from build123d import *

# Parameters (mm, degrees)
SKETCH1_W            = 914
SKETCH1_H            = 430
BOSS_EXTRUDE1_DEPTH  = 15
CUT_EXTRUDE2_DEPTH   = 16
LPATTERN1_COUNT      = 4
LPATTERN1_PITCH      = 80
MIRROR1_COPY_1_DEPTH = 16
MIRROR1_COPY_2_DEPTH = 16
MIRROR1_COPY_3_DEPTH = 16


with BuildPart() as part:
    # Sketch1 → Boss-Extrude1 (new body)
    with BuildSketch(Plane(origin=(0, 0, 0), x_dir=(1, 0, 0), z_dir=(0, 1, 0))):
        Rectangle(SKETCH1_W, SKETCH1_H)
    extrude(amount=BOSS_EXTRUDE1_DEPTH)

    # Sketch2 → Cut-Extrude2 (cut, through all)
    with BuildSketch(Plane(origin=(0, 15, 0), x_dir=(1, 0, 0), z_dir=(0, 1, 0))):
        with BuildLine():
            Line((364.726860249, -182.685298289), (381.301805569, -182.685298289))
            ThreePointArc((381.301805569, -182.685298289), (386.251553037, -180.635045758), (388.301805569, -175.685298289))
            Line((388.301805569, -175.685298289), (388.301805569, 175.685298289))
            ThreePointArc((388.301805569, 175.685298289), (386.251553037, 180.635045758), (381.301805569, 182.685298289))
            Line((381.301805569, 182.685298289), (364.726860249, 182.685298289))
            ThreePointArc((364.726860249, 182.685298289), (359.77711278, 180.635045758), (357.726860249, 175.685298289))
            Line((357.726860249, 175.685298289), (357.726860249, -175.685298289))
            ThreePointArc((357.726860249, -175.685298289), (359.77711278, -180.635045758), (364.726860249, -182.685298289))
        make_face()
    cut_extrude2 = extrude(amount=-CUT_EXTRUDE2_DEPTH, mode=Mode.SUBTRACT)

    # LPattern1: Cut-Extrude2 ×4
    with Locations(*[(-i * LPATTERN1_PITCH, 0, 0) for i in range(1, LPATTERN1_COUNT)]):
        add(cut_extrude2, mode=Mode.SUBTRACT)

    # Mirror1: Cut-Extrude2 across plane
    add(cut_extrude2.mirror(Plane(origin=(0, 0, 0), x_dir=(0, 0, 1), z_dir=(1, 0, 0))), mode=Mode.SUBTRACT)

    # Mirror1 copy 1 sketch → Mirror1 copy 1 (cut, through all)
    with BuildSketch(Plane(origin=(80, 15, 0), x_dir=(-1, 0, 0), z_dir=(0, 1, 0))):
        with BuildLine():
            Line((364.726860249, 182.685298289), (381.301805569, 182.685298289))
            ThreePointArc((381.301805569, 182.685298289), (386.251553037, 180.635045758), (388.301805569, 175.685298289))
            Line((388.301805569, 175.685298289), (388.301805569, -175.685298289))
            ThreePointArc((388.301805569, -175.685298289), (386.251553037, -180.635045758), (381.301805569, -182.685298289))
            Line((381.301805569, -182.685298289), (364.726860249, -182.685298289))
            ThreePointArc((364.726860249, -182.685298289), (359.77711278, -180.635045758), (357.726860249, -175.685298289))
            Line((357.726860249, -175.685298289), (357.726860249, 175.685298289))
            ThreePointArc((357.726860249, 175.685298289), (359.77711278, 180.635045758), (364.726860249, 182.685298289))
        make_face()
    extrude(amount=-MIRROR1_COPY_1_DEPTH, mode=Mode.SUBTRACT)

    # Mirror1 copy 2 sketch → Mirror1 copy 2 (cut, through all)
    with BuildSketch(Plane(origin=(160, 15, 0), x_dir=(-1, 0, 0), z_dir=(0, 1, 0))):
        with BuildLine():
            Line((364.726860249, 182.685298289), (381.301805569, 182.685298289))
            ThreePointArc((381.301805569, 182.685298289), (386.251553037, 180.635045758), (388.301805569, 175.685298289))
            Line((388.301805569, 175.685298289), (388.301805569, -175.685298289))
            ThreePointArc((388.301805569, -175.685298289), (386.251553037, -180.635045758), (381.301805569, -182.685298289))
            Line((381.301805569, -182.685298289), (364.726860249, -182.685298289))
            ThreePointArc((364.726860249, -182.685298289), (359.77711278, -180.635045758), (357.726860249, -175.685298289))
            Line((357.726860249, -175.685298289), (357.726860249, 175.685298289))
            ThreePointArc((357.726860249, 175.685298289), (359.77711278, 180.635045758), (364.726860249, 182.685298289))
        make_face()
    extrude(amount=-MIRROR1_COPY_2_DEPTH, mode=Mode.SUBTRACT)

    # Mirror1 copy 3 sketch → Mirror1 copy 3 (cut, through all)
    with BuildSketch(Plane(origin=(240, 15, 0), x_dir=(-1, 0, 0), z_dir=(0, 1, 0))):
        with BuildLine():
            Line((364.726860249, 182.685298289), (381.301805569, 182.685298289))
            ThreePointArc((381.301805569, 182.685298289), (386.251553037, 180.635045758), (388.301805569, 175.685298289))
            Line((388.301805569, 175.685298289), (388.301805569, -175.685298289))
            ThreePointArc((388.301805569, -175.685298289), (386.251553037, -180.635045758), (381.301805569, -182.685298289))
            Line((381.301805569, -182.685298289), (364.726860249, -182.685298289))
            ThreePointArc((364.726860249, -182.685298289), (359.77711278, -180.635045758), (357.726860249, -175.685298289))
            Line((357.726860249, -175.685298289), (357.726860249, 175.685298289))
            ThreePointArc((357.726860249, 175.685298289), (359.77711278, 180.635045758), (364.726860249, 182.685298289))
        make_face()
    extrude(amount=-MIRROR1_COPY_3_DEPTH, mode=Mode.SUBTRACT)


solid = part.part
Input: part model. Units: mm. Frame: model coordinates. Give positions to 0.01 mm unless a question says otherwise; leave off trailing zeros. Use CSV: the item, a comma, the result in double quotes. Start each with the question number.
Item 1: Line query: line 1 (Z direction, x = -302.5, y = 6.25); line 2 (Z direction, x = -208, y = 13.5). Output: solid intervals per line, ascending.
Item 2: Contact query for a flat-ended pin moving along its axis: P1, Ø10, axis at x = -348, z = -26, coming from the -Y side. Output: stop coordinate, or through.
Item 3: Section A-A on z = 21. State how many separate pieces and enclosed holes the cut face has, then the cut area to 3 significant figures.
Ans:
1,line 1,"z = -215 to -182.58, 182.58 to 215"
1,line 2,"z = -215 to -182.69, 182.69 to 215"
2,P1,"stops at y = 0"
3,separate pieces,"9"
3,enclosed holes,"0"
3,area,"10,000 mm2"
